from build123d import *

# Parameters (mm, degrees)
BOSS_EXTRUDE1_DEPTH      = 2
BOSS_EXTRUDE2_DEPTH      = 1
SKETCH3_R                = 1
CUT_EXTRUDE1_DEPTH       = 1
BOSS_EXTRUDE3_DEPTH      = 2
BOSS_EXTRUDE3_DEPTH_BACK = 1
BOSS_EXTRUDE4_START      = -3
BOSS_EXTRUDE4_OUTLINE_R  = 1
BOSS_EXTRUDE4_DEPTH      = 3
SKETCH6_R                = 3.500627768
BOSS_EXTRUDE5_DEPTH      = 3
BOSS_EXTRUDE6_DEPTH      = 3
CUT_EXTRUDE2_DEPTH       = 15
FILLET1_R                = 20
FILLET2_R                = 3
FILLET3_R                = 3
SKETCH9_R                = 1
CUT_EXTRUDE3_DEPTH       = 15
CUT_EXTRUDE4_DEPTH       = 1.5
FILLET4_R                = 8
FILLET5_R                = 2
SKETCH11_W               = 110.258684369
SKETCH11_H               = 6.064888907
CUT_EXTRUDE5_DEPTH       = 38
SKETCH12_R               = 18.613151801
CUT_EXTRUDE6_DEPTH       = 29
SKETCH13_W               = 77.706478895
SKETCH13_H               = 41.021519778
CUT_EXTRUDE7_DEPTH       = 1
FILLET6_START            = -4.447684996
FILLET6_DEPTH            = 2
FILLET6_START_2          = 2.447684996
FILLET6_2_DEPTH          = 2
FILLET6_START_3          = -1
FILLET6_3_DEPTH          = 1
FILLET6_START_4          = -2.447684996
FILLET6_4_DEPTH          = 4.895369992


with BuildPart() as part:
    # Sketch1 → Boss-Extrude1 (new body)
    with BuildSketch(Plane.XY):
        with BuildLine():
            Line((14.458185053, 3.677415528), (0.579181495, 5.217954465))
            ThreePointArc((0.579181495, 5.217954465), (-5.25, 0), (0.579181495, -5.217954465))
            Line((0.579181495, -5.217954465), (14.458185053, -3.677415528))
            ThreePointArc((14.458185053, -3.677415528), (17.75, 0), (14.458185053, 3.677415528))
        make_face()
        with BuildLine():
            Line((14.292704626, 2.186571395), (0.413701068, 3.727110332))
            ThreePointArc((0.413701068, 3.727110332), (-3.75, 0), (0.413701068, -3.727110332))
            Line((0.413701068, -3.727110332), (14.292704626, -2.186571395))
            ThreePointArc((14.292704626, -2.186571395), (16.25, 0), (14.292704626, 2.186571395))
        make_face(mode=Mode.SUBTRACT)
    extrude(amount=BOSS_EXTRUDE1_DEPTH)

    # Sketch2 → Boss-Extrude2 (add)
    with BuildSketch(Plane.XY.offset(2)):
        with BuildLine():
            Line((14.458185053, 3.677415528), (0.579181495, 5.217954465))
            ThreePointArc((0.579181495, 5.217954465), (-5.25, 0), (0.579181495, -5.217954465))
            Line((0.579181495, -5.217954465), (14.458185053, -3.677415528))
            ThreePointArc((14.458185053, -3.677415528), (17.75, 0), (14.458185053, 3.677415528))
        make_face()
    extrude(amount=BOSS_EXTRUDE2_DEPTH)

    # Sketch3 → Cut-Extrude1 (cut)
    with BuildSketch(Plane.XY.offset(3)):
        Circle(SKETCH3_R)
    extrude(amount=-CUT_EXTRUDE1_DEPTH, mode=Mode.SUBTRACT)

    # Sketch4 → Boss-Extrude3 (add, two sides: drawn at the far end of the back side and taken through both)
    with BuildSketch(Plane(origin=(0, 0, 2), x_dir=(-1, 0, 0), z_dir=(0, 0, -1)).offset(-BOSS_EXTRUDE3_DEPTH_BACK)):
        with BuildLine():
            Line((-15.26072202, 2.426182253), (-7.518683274, 4.447684996))
            Line((-7.518683274, 4.447684996), (-42.518683274, 4.447684996))
            ThreePointArc((-42.518683274, 4.447684996), (-39.373695053, 3.144988221), (-38.070998278, 0))
            ThreePointArc((-38.070998278, 0), (-39.373695053, -3.144988221), (-42.518683274, -4.447684996))
            Line((-42.518683274, -4.447684996), (-7.518683274, -4.447684996))
            Line((-7.518683274, -4.447684996), (-13.862339481, -2.595687971))
            Line((-13.862339481, -2.595687971), (-16.213670101, -1.84565397))
            Line((-16.213670101, -1.84565397), (-17.166618181, 0))
            Line((-17.166618181, 0), (-15.26072202, 2.426182253))
        make_face()
        with BuildLine():
            ThreePointArc((-38.070998278, 0), (-39.373695053, 3.144988221), (-42.518683274, 4.447684996))
            Line((-42.518683274, 4.447684996), (-42.518683274, 2))
            ThreePointArc((-42.518683274, 2), (-41.104469712, 1.414213562), (-40.518683274, 0))
            ThreePointArc((-40.518683274, 0), (-41.104469712, -1.414213562), (-42.518683274, -2))
            Line((-42.518683274, -2), (-42.518683274, -4.447684996))
            ThreePointArc((-42.518683274, -4.447684996), (-39.373695053, -3.144988221), (-38.070998278, 0))
        make_face()
        with BuildLine():
            Line((-42.518683274, 2), (-42.518683274, 4.447684996))
            ThreePointArc((-42.518683274, 4.447684996), (-46.96636827, 0), (-42.518683274, -4.447684996))
            Line((-42.518683274, -4.447684996), (-42.518683274, -2))
            ThreePointArc((-42.518683274, -2), (-44.518683274, 0), (-42.518683274, 2))
        make_face()
    extrude(amount=BOSS_EXTRUDE3_DEPTH + BOSS_EXTRUDE3_DEPTH_BACK)

    # Boss-Extrude4: read off the stored shape, not the designer's step
    # Boss-Extrude4 outline → Boss-Extrude4 (add)
    with BuildSketch(Plane(origin=(0, 0, 0), x_dir=(-1, 0, 0), z_dir=(0, 0, -1)).offset(BOSS_EXTRUDE4_START)):
        with BuildLine():
            ThreePointArc((-42.518683274, -4.447684996), (-46.96636827, 0), (-42.518683274, 4.447684996))
            Line((-42.518683274, 4.447684996), (-54.290526798, 4.447684996))
            ThreePointArc((-54.290526798, 4.447684996), (-59.289068337, 5.305033813), (-63.716210719, 7.779073998))
            ThreePointArc((-63.716210719, 7.779073998), (-80, 0), (-63.716210719, -7.779073998))
            ThreePointArc((-63.716210719, -7.779073998), (-59.289068337, -5.305033813), (-54.290526798, -4.447684996))
            Line((-54.290526798, -4.447684996), (-42.518683274, -4.447684996))
        make_face()
        with Locations((-68.205771366, -4.5)):
            Circle(BOSS_EXTRUDE4_OUTLINE_R, mode=Mode.SUBTRACT)
        with Locations((-76, 0)):
            Circle(BOSS_EXTRUDE4_OUTLINE_R, mode=Mode.SUBTRACT)
        with Locations((-68.205771366, 4.5)):
            Circle(BOSS_EXTRUDE4_OUTLINE_R, mode=Mode.SUBTRACT)
    extrude(amount=BOSS_EXTRUDE4_DEPTH)

    # Sketch6 → Boss-Extrude5 (add)
    with BuildSketch(Plane(origin=(0, 0, 0), x_dir=(-1, 0, 0), z_dir=(0, 0, -1))):
        with Locations((-42.518683274, 0)):
            Circle(SKETCH6_R)
    extrude(amount=-BOSS_EXTRUDE5_DEPTH)

    # Sketch7 → Boss-Extrude6 (add)
    with BuildSketch(Plane(origin=(0, 0, 0), x_dir=(-1, 0, 0), z_dir=(0, 0, -1))):
        Polygon((-54.290526798, 4.447684996), (-94.290526798, 4.447684996), (-94.290526798, -3.552315004), (-68.73970048, -3.552315004), (-92.931542949, -17.519481766), (-88.931542949, -24.447684996), (-54.290526798, -4.447684996), align=None)
    extrude(amount=-BOSS_EXTRUDE6_DEPTH)

    # Sketch8 → Cut-Extrude2 (cut)
    with BuildSketch(Plane(origin=(0, 0, 0), x_dir=(-1, 0, 0), z_dir=(0, 0, -1))):
        Polygon((-94.290526798, 4.447684996), (-45.837456427, 4.447684996), (-68.326886593, 15.265325323), align=None)
        Polygon((-94.290526798, -3.552315004), (-68.73970048, -3.552315004), (-92.931542949, -17.519481766), align=None)
    extrude(amount=-CUT_EXTRUDE2_DEPTH, mode=Mode.SUBTRACT)

    # Fillet1
    fillet1_edges = [part.edges().sort_by_distance(p)[0] for p in [
        (54.290526798, -4.447684996, 1.5),
    ]]
    fillet(fillet1_edges, radius=FILLET1_R)

    # Fillet2
    fillet2_edges = [part.edges().sort_by_distance(p)[0] for p in [
        (94.290526798, 4.447684996, 1.5),
        (94.290526798, -3.552315004, 1.5),
        (92.931542949, -17.519481766, 1.5),
        (88.931542949, -24.447684996, 1.5),
    ]]
    fillet(fillet2_edges, radius=FILLET2_R)

    # Fillet3
    fillet3_edges = [part.edges().sort_by_distance(p)[0] for p in [
        (68.73970048, -3.552315004, 1.5),
    ]]
    fillet(fillet3_edges, radius=FILLET3_R)

    # Sketch9 → Cut-Extrude3 (cut)
    with BuildSketch(Plane(origin=(0, 0, 0), x_dir=(-1, 0, 0), z_dir=(0, 0, -1))):
        with Locations((-89.290526798, 0.447684996)):
            Circle(SKETCH9_R)
        with Locations((-79.290526798, 0.447684996)):
            Circle(SKETCH9_R)
        with Locations((-77.941161892, -13.483583381)):
            Circle(SKETCH9_R)
        with Locations((-86.60141593, -18.483583381)):
            Circle(SKETCH9_R)
    extrude(amount=-CUT_EXTRUDE3_DEPTH, mode=Mode.SUBTRACT)

    # Sketch10 → Cut-Extrude4 (cut)
    with BuildSketch(Plane(origin=(0, 0, 0), x_dir=(-1, 0, 0), z_dir=(0, 0, -1))):
        with BuildLine():
            Line((-19.05, 2.447684996), (-67.154630008, 2.447684996))
            ThreePointArc((-67.154630008, 2.447684996), (-70.616179326, -5.909234314), (-62.259260015, -2.447684996))
            Line((-62.259260015, -2.447684996), (-19.05, -2.447684996))
            Line((-19.05, -2.447684996), (-19.05, 2.447684996))
        make_face()
    extrude(amount=-CUT_EXTRUDE4_DEPTH, mode=Mode.SUBTRACT)

    # Fillet4
    fillet4_edges = [part.edges().sort_by_distance(p)[0] for p in [
        (62.259260015, -2.447684996, 0.75),
    ]]
    fillet(fillet4_edges, radius=FILLET4_R)

    # Fillet5
    fillet5_edges = [part.edges().sort_by_distance(p)[0] for p in [
        (19.05, 2.447684996, 0.75),
        (19.05, -2.447684996, 0.75),
    ]]
    fillet(fillet5_edges, radius=FILLET5_R)

    # Mirror1: part across plane


with BuildPart() as part_1:
    add(part.part)
    add(part.part.mirror(Plane(origin=(14.05, 0, 0), x_dir=(1, 0, 0), z_dir=(0, 0, 1))))

    # Sketch11 → Cut-Extrude5 (cut)
    with BuildSketch(Plane(origin=(0, 4.447684996, 0), x_dir=(1, 0, 0), z_dir=(0, 1, 0))):
        with Locations((47.771534573, -3.032444454)):
            Rectangle(SKETCH11_W, SKETCH11_H)
    extrude(amount=-CUT_EXTRUDE5_DEPTH, mode=Mode.SUBTRACT)

    # Sketch12 → Cut-Extrude6 (cut)
    with BuildSketch(Plane.XY):
        with Locations((7.534351793, 3.599902348)):
            Circle(SKETCH12_R)
    extrude(amount=CUT_EXTRUDE6_DEPTH, mode=Mode.SUBTRACT)

    # Sketch13 → Cut-Extrude7 (cut)
    with BuildSketch(Plane.XY):
        with Locations((57.903239447, -8.718962854)):
            Rectangle(SKETCH13_W, SKETCH13_H)
    extrude(amount=-CUT_EXTRUDE7_DEPTH, mode=Mode.SUBTRACT)

    # Fillet6: read off the stored shape, not the designer's step
    # Fillet6 outline → Fillet6 (add)
    with BuildSketch(Plane(origin=(0, 0, 0), x_dir=(1, 0, 0), z_dir=(0, 1, 0)).offset(FILLET6_START)):
        with BuildLine():
            Line((19.05, 1), (19.049997006, -1.45e-06))
            ThreePointArc((19.049997006, -1.45e-06), (21.172829345, 0.746793973), (23.408898944, 1))
            Line((23.408898944, 1), (19.05, 1))
        make_face()
    extrude(amount=FILLET6_DEPTH)

    # Fillet6 2 outline → Fillet6 2 (add)
    with BuildSketch(Plane(origin=(0, 0, 0), x_dir=(1, 0, 0), z_dir=(0, 1, 0)).offset(FILLET6_START_2)):
        with BuildLine():
            Line((19.05, 1), (19.049997006, -1.45e-06))
            ThreePointArc((19.049997006, -1.45e-06), (21.172829345, 0.746793973), (23.408898944, 1))
            Line((23.408898944, 1), (19.05, 1))
        make_face()
    extrude(amount=FILLET6_2_DEPTH)

    # Fillet6 3 outline → Fillet6 3 (add)
    with BuildSketch(Plane.XY.offset(FILLET6_START_3)):
        with BuildLine():
            Line((19.05, 2.447684996), (19.05, 0.447684996))
            ThreePointArc((19.05, 0.447684996), (19.635786438, 1.861898559), (21.05, 2.447684996))
            Line((21.05, 2.447684996), (19.05, 2.447684996))
        make_face()
        with BuildLine():
            ThreePointArc((21.05, -2.447684996), (19.635786438, -1.861898559), (19.05, -0.447684996))
            Line((19.05, -0.447684996), (19.05, -2.447684996))
            Line((19.05, -2.447684996), (21.05, -2.447684996))
        make_face()
    extrude(amount=FILLET6_3_DEPTH)

    # Fillet6 4 outline → Fillet6 4 (cut)
    with BuildSketch(Plane(origin=(0, 0, 0), x_dir=(1, 0, 0), z_dir=(0, 1, 0)).offset(FILLET6_START_4)):
        with BuildLine():
            ThreePointArc((23, 0.991636585), (20.973982557, 0.699029961), (19.049997006, -1.45e-06))
            Line((19.049997006, -1.45e-06), (18, -0.508538641))
            Line((18, -0.508538641), (18, -1))
            Line((18, -1), (23, -1))
            Line((23, -1), (23, 0.991636585))
        make_face()
    extrude(amount=FILLET6_4_DEPTH, mode=Mode.SUBTRACT)


solid = part_1.part
The listing builds one solid part. Answer for the finished solid, in the listing's coordinates (mm). A direction names the side the tool comes from. Coordinates: 2 decimals unless noted, no trailing zeros. Write each loop counter-clockwise with the first axis right and the second up, starting at its lowest first coordinate (ties: lowest second). Pieces come first, ordered by that corner, then holes. Notation, with made-up numbers: M 15.5,-24 L 27.5,-24 A14 ccw 27.5,-14 Z; hole C -22,33 d5. An arc over 180 degrees is marked long. Put each result on its own line as item: value. Start each with the question number.
1. Consider line 1 (Y direction, x = 0, z = -2.2); line 2 (Y direction, x = 39.5, z = -1.2); line 3 (Z direction, x = 77, y = -11.25). Determine where each line is inside the solid, lowest interval first. Write a range as from..to.
2. For a pull along X with two mould halves and no side action, classify faces 1 (the flat face through (49, 4.448, -2)), 2 (the flat face through (94.291, 0, -2)), 3 (the cylindrical face through (54, -5.1, -2)), 4 (the cylindrical face through (71.6, -4.5, -1.2)) as pulls with the +X half, pulls with the -X half, needs draft (parallel to the pull), parting line crosses it, or undercut.
3. Which of the six approach directions +Z, -Z, +X, -X, +Y, -Y give full straight-line access (tool end or side, diameter ignored) to faces 5 (the flat face through (4, -4.84, -1.48)), 6 (the flat face through (7, 4, 0)), 7 (the flat face through (4.098, 4.827, -1.479)), 8 (the cylindrical face through (-3.75, 0.09, -0.99)), 9 (the flat face through (86, -3.552, -2))?
4. A cutting plane is placed at B-B on y = -21. Write down the section's boundary in (x, z).
5. A cutting plane is placed at A-A on x = 47. Write down the section's boundary in (y, z).
6. Flat-ended cylindrical pins translate along their axes: P1, Ø1.5, axis at x = 33, z = -2, coming from the -Y side; P2, Ø5, axis at x = 72.5, y = -15.5, coming from the +Z side; P3, Ø1.6, axis at x = 85.5, z = -1.5, coming from the -Y side; P4, Ø1.8, axis at x = 86.6, y = -18.48, coming from the +Z side. Find the tip coordinate at first contact, or state that the pin passes through.
7. A cutting plane is placed at C-C on y = -11.5. Write down the section's boundary in (x, z), then the cut area to 3 significant figures.
Resolved:
1. line 1: y = -5.25..-1, 1..5.25
1. line 2: y = -4.45..-2.45, 2.45..4.45
1. line 3: z = -3..-1
2. face 1: needs draft
2. face 2: pulls with the +X half
2. face 3: undercut
2. face 4: undercut
3. face 5: +Z, -Z, -Y
3. face 6: +Z, +X, -X, +Y, -Y
3. face 7: +Z, -Z, +X, +Y
3. face 8: +Z
3. face 9: +Z, -Z, +X
4. outline: M 82.96,-3 L 90.92,-3 L 90.92,-1 L 82.96,-1 Z
5. outline: M -4.45,-3 L 4.45,-3 L 4.45,-1 L 2.45,-1 L 2.45,-1.5 L -2.45,-1.5 L -2.45,-1 L -4.45,-1 Z
6. P1: stops at y = -4.45
6. P2: stops at z = -1
6. P3: stops at y = -22.93
6. P4: passes through
7. outline: M 66.51,-3 L 82.51,-3 L 82.51,-1 L 66.51,-1 Z
7. area: 32.0 mm2
